The model under review builds one solid part; all positions refer to its coordinate system, in mm. Coordinates: 2 decimals unless noted, no trailing zeros. Order: outer loops, then holes, each group sorted by start corner. A loop starts at its lowest first (then second) coordinate and runs counter-clockwise, first axis right, second up. Notation, with made-up numbers: M 41.25,-1.75 L 52.25,-1.75 A3 ccw 52.25,2.25 Z; hole C 73,-19.75 d3. An arc over 180 degrees is marked long. Answer as CSV lines item,"result". Start each with the question number.
Q1. For P1, Ø1.5, axis at y = 1.5, z = 54, coming from the +X side; P2, Ø0.9, axis at y = 1, z = 35.5, coming from the +X side; P3, Ø0.9, axis at x = -45.5, y = 2, coming from the -Z side; P4, Ø1.5, axis at x = -60, z = -68.5, coming from the -Y side (3 decimals), all flat-tipped, find the tip position at first contact; note any pin that passes through.
Q2. Consider section B-B on z = -25.5. Write out the cut boundary in (x, y), and give its area (3 significant figures).
Q3. Consider section C-C on y = 1.45. State how many separate pieces and enclosed holes the cut face has, and give its area (3 significant figures).
Q4. Consider section A-A on x = -47. Write out the cut boundary in (y, z), and give its area (3 significant figures).
Q5. Consider section D-D on z = -51. Write out the cut boundary in (x, y), and give its area (3 significant figures).
Q6. Wall thickness on L1, parallel to X at y = 2.05, z = -26; L2, parallel to Z at x = 49, y = 2.35; L3, parallel to X at y = 2.15, z = 5: over which ranges is each line inside the solid? List them lowest first. Write a range as [from, to].
Autodesk Inventor part; units mm, degrees
ref_plane "YZ Plane" through (0, 0, 0) normal (1, 0, 0) x (0, 1, 0)
ref_plane "XZ Plane" through (0, 0, 0) normal (0, 1, 0) x (-1, 0, 0)
ref_plane "XY Plane" through (0, 0, 0) normal (0, 0, 1) x (1, 0, 0)
sketch "Sketch1" plane through (0, 0, 0) normal (0, 1, 0) x (-1, 0, 0)
  circle A0 centre (0, 0) radius 90
  line L0 (-71.239, 55) -> (71.239, 55)
  dimension "d0" = 180
  dimension "d1" = 55
extrude "Extrusion1" add sketch "Sketch1" along normal blind 3 contours A0 L0 picked at (-1.0947, 6.6866)
sketch "Sketch2" plane through (0, 3, 0) normal (0, 1, 0) x (1, 0, 0)
  line L0 (-71.239, -55) -> (71.239, -55)
  line L1 (-70, -55) -> (-60, -55)
  line L2 (-60, -55) -> (-60, -52)
  line L3 (-60, -52) -> (-70, -52)
  line L4 (-70, -52) -> (-70, -55)
  line L5 (-30, -55) -> (-10, -55)
  line L6 (-10, -55) -> (-10, -52)
  line L7 (-10, -52) -> (-30, -52)
  line L8 (-30, -52) -> (-30, -55)
  point P0 (0, 0)
  dimension "d4" = 10
  dimension "d5" = 3
  dimension "d6" = 20
  dimension "d7" = 3
  dimension "d8" = 10
  dimension "d9" = 30
extrude "Extrusion2" cut sketch "Sketch2" against normal blind 3
sketch "Sketch3" plane through (0, 3, 0) normal (0, 1, 0) x (1, 0, 0)
  line L0 (-57, -42) -> (-60, -42)
  line L1 (-60, -42) -> (-60, -22)
  line L2 (-60, -22) -> (-57, -22)
  line L3 (-57, -22) -> (-57, -42)
  line L4 (-57, -12) -> (-60, -12)
  line L5 (-60, -12) -> (-60, -2)
  line L6 (-60, -2) -> (-57, -2)
  line L7 (-57, -2) -> (-57, -12)
  line L8 (-57, 18) -> (-60, 18)
  line L9 (-60, 18) -> (-60, 38)
  line L10 (-60, 38) -> (-57, 38)
  line L11 (-57, 38) -> (-57, 18)
  line L12 (-70, -52) -> (-60, -52)
  point P0 (0, 0)
  dimension "d12" = 3
  dimension "d13" = 20
  dimension "d14" = 3
  dimension "d15" = 10
  dimension "d16" = 3
  dimension "d17" = 20
  dimension "d18" = 10
  dimension "d19" = 10
  dimension "d20" = 20
  dimension "d21" = 57
extrude "Extrusion3" cut sketch "Sketch3" against normal blind 3
sketch "Sketch4" plane through (0, 3, 0) normal (0, 1, 0) x (1, 0, 0)
  line L0 (-42.5, -34) -> (-52.5, -34)
  line L1 (-52.5, -34) -> (-52.5, -37)
  line L2 (-52.5, -37) -> (-42.5, -37)
  line L3 (-42.5, -37) -> (-42.5, -34)
  line L4 (-42.5, 14) -> (-52.5, 14)
  line L5 (-52.5, 14) -> (-52.5, 11)
  line L6 (-52.5, 11) -> (-42.5, 11)
  line L7 (-42.5, 11) -> (-42.5, 14)
  line L8 (-70, -52) -> (-60, -52)
  line L9 (-57, -22) -> (-57, -42)
  point P0 (0, 0)
  dimension "d24" = 10
  dimension "d25" = 3
  dimension "d26" = 10
  dimension "d27" = 3
  dimension "d28" = 15
  dimension "d29" = 45
  dimension "d30" = 4.5
extrude "Extrusion4" cut sketch "Sketch4" against normal blind 3
mirror "Mirror1" about plane through (0, 0, 0) normal (1, 0, 0) of "Extrusion4", "Extrusion3", "Extrusion2"
properties part number "Top Plate"
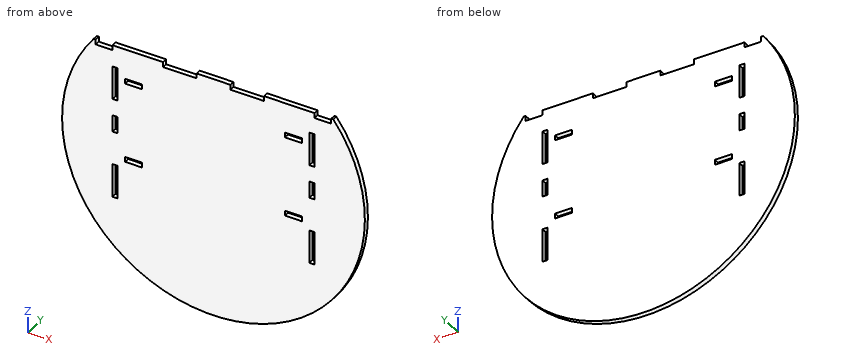
Evaluation:
1,P1,"stops at x = 72.56"
1,P2,"stops at x = 82.89"
1,P3,"stops at z = -77.91"
1,P4,"passes through"
2,outline,"M -86.31,0 L -60,0 L -60,3 L -86.31,3 Z; M -57,0 L 57,0 L 57,3 L -57,3 Z; M 60,0 L 86.31,0 L 86.31,3 L 60,3 Z"
2,area,"500 mm²"
3,separate pieces,"1"
3,enclosed holes,"10"
3,area,"21,400 mm²"
4,outline,"M 0,-76.75 L 3,-76.75 L 3,-14 L 0,-14 Z; M 0,-11 L 3,-11 L 3,34 L 0,34 Z; M 0,37 L 3,37 L 3,55 L 0,55 Z"
4,area,"377 mm²"
5,outline,"M -74.16,0 L 74.16,0 L 74.16,3 L -74.16,3 Z"
5,area,"445 mm²"
6,L1,"x = [-86.16, -60], [-57, 57], [60, 86.16]"
6,L2,"z = [-75.49, -14], [-11, 34], [37, 55]"
6,L3,"x = [-89.86, -60], [-57, 57], [60, 89.86]"
